For this review, take the finished solid that the model builds, in its own axes (mm). A direction names the side the tool comes from. Round coordinates to 2 decimals unless told otherwise and drop trailing zeros. Order: outer loops, then holes, each group sorted by start corner. A loop starts at its lowest first (then second) coordinate and runs counter-clockwise, first axis right, second up. Notation, with made-up numbers: M 37,83.5 L 74,83.5 A33 ccw 74,122.5 Z; hole C -20,65 d8. An arc over 180 degrees is marked long. Answer as a JSON object with one key per item and string values.
from build123d import *

# Parameters (mm, degrees)
SKETCH1_R                = 19.5
SKETCH1_R_2              = 18
BOSS_EXTRUDE1_DEPTH      = 34
BOSS_EXTRUDE2_DEPTH      = 4.9
BOSS_EXTRUDE2_DEPTH_BACK = 52.1
SKETCH2_R                = 18
SKETCH3_R                = 6.5
BOSS_EXTRUDE3_DEPTH      = 4.5
SKETCH4_R                = 1.585
BOSS_EXTRUDE4_DEPTH      = 11
SKETCH5_W                = 0.5
SKETCH5_H                = 4.75
BOSS_EXTRUDE5_DEPTH      = 7.4


with BuildPart() as part:
    # Sketch1 → Boss-Extrude1 (new body)
    with BuildSketch(Plane(origin=(0, 0, 0), x_dir=(1, 0, 0), z_dir=(0, 1, 0))):
        with Locations(Location((0, 0, 0), (0, 0, 270))):
            Circle(SKETCH1_R)
        with Locations(Location((0, 0, 0), (0, 0, 270))):
            Circle(SKETCH1_R_2, mode=Mode.SUBTRACT)
    extrude(amount=BOSS_EXTRUDE1_DEPTH)

    # Sketch2 → Boss-Extrude2 (add, two sides: drawn at the far end of the back side and taken through both)
    with BuildSketch(Plane(origin=(0, 34, 0), x_dir=(1, 0, 0), z_dir=(0, 1, 0)).offset(-BOSS_EXTRUDE2_DEPTH_BACK)):
        with Locations(Location((0, 0, 0), (0, 0, 270))):
            Circle(SKETCH2_R)
    extrude(amount=BOSS_EXTRUDE2_DEPTH + BOSS_EXTRUDE2_DEPTH_BACK)

    # Sketch3 → Boss-Extrude3 (add)
    with BuildSketch(Plane(origin=(0, 38.9, 0), x_dir=(1, 0, 0), z_dir=(0, 1, 0))):
        with Locations(Location((0, 0, 0), (0, 0, 270))):
            Circle(SKETCH3_R)
    extrude(amount=BOSS_EXTRUDE3_DEPTH)

    # Sketch4 → Boss-Extrude4 (add)
    with BuildSketch(Plane(origin=(0, 43.4, 0), x_dir=(1, 0, 0), z_dir=(0, 1, 0))):
        with Locations(Location((0, 0, 0), (0, 0, 270))):
            Circle(SKETCH4_R)
    extrude(amount=BOSS_EXTRUDE4_DEPTH)

    # Sketch5 → Boss-Extrude5 (add)
    with BuildSketch(Plane.XZ.offset(18.1)):
        with Locations((14.75, 0)):
            Rectangle(SKETCH5_W, SKETCH5_H)
        with Locations((-14.75, 0)):
            Rectangle(SKETCH5_W, SKETCH5_H)
    extrude(amount=BOSS_EXTRUDE5_DEPTH)


solid = part.part
1) Machinability: for faces 5 (the flat face through (14.5, -22, 0)), 6 (the flat face through (-15, -22, 0)), 7 (the cylindrical face through (-0.96, 48.82, -1.26)), 8 (the cylindrical face through (5.407, -9.177, 17.169)), 9 (the cylindrical face through (19.334, 16.762, -2.539)), which of the approach directions +Z, -Z, +X, -X, +Y, -Y give a long, thin tool a straight path to every point of the face, cutting with its end or side? Answer none if there is none.
Geometry check:
{"face 5": "+Z, -Z, -Y", "face 6": "+Z, -Z, -X, -Y", "face 7": "+Y", "face 8": "-Y", "face 9": "+Y, -Y"}
2) Insertion check: P1, Ø2, axis at x = -1.5, y = 16, coming from the +Z side; P2, Ø5, axis at x = 4.5, y = 44.5, coming from the -Z side; P3, Ø6, axis at x = -11.5, z = 2, coming from the +Y side. Each pin has a flat end and moves straight along its axis. Give the tip position at first contact, or say it passes through.
Geometry check:
{"P1": "stops at z = 19.49", "P2": "stops at z = -6.1", "P3": "stops at y = 38.9"}
3) Add section D-D on z = 8. State the section outline as (x, y) points, and give its area (3 significant figures).
Geometry check:
{"outline": "M -17.78,0 L -16.12,0 L -16.12,-18.1 L 16.12,-18.1 L 16.12,0 L 17.78,0 L 17.78,34 L 16.12,34 L 16.12,38.9 L -16.12,38.9 L -16.12,34 L -17.78,34 Z", "area": "1,950 mm²"}
4) Add section C-C on y = 37.5. State the section outline as (x, z) points, and give its area (3 significant figures).
Geometry check:
{"outline": "C 0,0 d36", "area": "1,020 mm²"}
5) Add section A-A on z = 0. State the section outline as (x, y) points (3 decimals), and give its area (3 significant figures).
Geometry check:
{"outline": "M -19.5,0 L -18,0 L -18,-18.1 L -15,-18.1 L -15,-25.5 L -14.5,-25.5 L -14.5,-18.1 L 14.5,-18.1 L 14.5,-25.5 L 15,-25.5 L 15,-18.1 L 18,-18.1 L 18,0 L 19.5,0 L 19.5,34 L 18,34 L 18,38.9 L 6.5,38.9 L 6.5,43.4 L 1.585,43.4 L 1.585,54.4 L -1.585,54.4 L -1.585,43.4 L -6.5,43.4 L -6.5,38.9 L -18,38.9 L -18,34 L -19.5,34 Z", "area": "2,250 mm²"}
6) Add section B-B on x = -4.5. State the section outline as (y, z) points, and give its area (3 significant figures).
Geometry check:
{"outline": "M -18.1,-17.43 L 0,-17.43 L 0,-18.97 L 34,-18.97 L 34,-17.43 L 38.9,-17.43 L 38.9,-4.69 L 43.4,-4.69 L 43.4,4.69 L 38.9,4.69 L 38.9,17.43 L 34,17.43 L 34,18.97 L 0,18.97 L 0,17.43 L -18.1,17.43 Z", "area": "2,130 mm²"}
7) For L1, parallel to Y at x = -11, z = -5; L2, parallel to Y at x = 5, z = 0; L3, parallel to Z at x = 6, y = 25, list the stretches that pass through material, from the lowest coordinate up.
Geometry check:
{"L1": "y = -18.1 to 38.9", "L2": "y = -18.1 to 43.4", "L3": "z = -18.55 to 18.55"}
8) Mouldability with a two-part tool opening along X and no side actions: class faces 1 (the flat face through (-17.24, 0, 5.69)), 2 (the cylindrical face through (-3.955, 41.118, -5.158)), 3 (the flat face through (-14.5, -22, 0)), 4 (the flat face through (15, -22, 0)) as +X half, -X half, draft (parallel to the pull), parting line (faces both ways), or undercut.
Geometry check:
{"face 1": "draft", "face 2": "parting line", "face 3": "undercut", "face 4": "+X half"}
